from build123d import *


with BuildPart() as part:
    # Sketch6 → Revolve1 (revolve)
    with BuildSketch(Plane.XY, mode=Mode.PRIVATE) as revolve1_sk:
        with BuildLine():
            Line((50.8, 22.53035676), (50.8, 6.35))
            Line((50.8, 6.35), (53.975, 6.35))
            Line((53.975, 6.35), (53.975, 20.227565916))
            add(Edge.make_bspline(
                [(53.975, 20.227565916), (54.291634879, 20.330430839), (55.162475518, 20.612719168), (56.636149311, 21.087725347), (58.867170376, 21.80102074), (61.522421046, 22.638682883), (64.736507837, 23.637812157), (68.023541536, 24.646609183), (72.39438926, 25.969741612), (77.802325895, 27.573199633), (84.37229967, 29.477097548), (93.118193973, 31.954107645), (108.466778526, 36.165197289), (130.491628823, 41.875745108), (165.870302673, 50.489926314), (210.303076361, 60.449379541), (281.693068548, 75.067985253), (371.347473816, 91.310304544), (479.374979471, 108.229836311), (569.684892552, 120.376775068), (642.076792345, 128.912483065), (696.438363769, 134.692640498), (750.863527692, 139.800693107), (796.267539796, 143.42521879), (832.617797313, 145.860290015), (859.890749047, 147.416222506), (882.628689993, 148.436275801), (898.53412358, 148.946546098), (907.62769622, 149.150954449), (912.14731785, 149.217348506), (914.4107585, 149.225018228)],
                knots=[0.06148136, 0.06148136, 0.06148136, 0.06148136, 0.06256458, 0.064402689, 0.066240798, 0.069917015, 0.073593232, 0.07726945, 0.080945667, 0.088298102, 0.095650536, 0.103002971, 0.11770784, 0.147117579, 0.176527318, 0.235346795, 0.294166272, 0.411805227, 0.529444182, 0.647083136, 0.705902613, 0.764722091, 0.823541568, 0.882361045, 0.911770784, 0.941180523, 0.970590261, 0.985295131, 0.992647565, 1, 1, 1, 1], degree=3))
            Line((914.4107585, 149.225018228), (914.4107585, 146.05))
            Line((914.4107585, 146.05), (1066.8, 146.05))
            Line((1066.8, 146.05), (1066.8, 149.225))
            Line((1066.8, 149.225), (965.2, 149.225))
            Line((965.2, 149.225), (965.2, 152.4))
            Line((965.2, 152.4), (914.4, 152.4))
            add(Edge.make_bspline(
                [(50.8, 22.53035676), (51.62596102, 22.801930188), (53.247366667, 23.331443773), (57.113810342, 24.581671091), (62.137627853, 26.163245596), (68.472923462, 28.113411094), (76.389796689, 30.474842786), (85.386033894, 33.081102875), (95.241355255, 35.841520364), (106.104903016, 38.788706559), (117.812200959, 41.867831442), (130.423899043, 45.08497442), (143.907449646, 48.417167108), (158.285989872, 51.860839853), (172.682057827, 55.208017205), (187.101006341, 58.468808185), (201.536340401, 61.648015415), (215.98908439, 64.751824582), (234.073297096, 68.542392147), (255.802551989, 72.956576003), (281.189453131, 77.92470015), (306.614812158, 82.692611325), (328.432361696, 86.646151134), (350.268122203, 90.497714312), (372.121192631, 94.250003895), (397.640090518, 98.488121242), (426.834492226, 103.147632175), (456.056824987, 107.628600482), (485.305388678, 111.934967932), (514.578772116, 116.069226586), (543.875783343, 120.032588186), (573.19542697, 123.82488003), (602.536868801, 127.444739672), (631.89942018, 130.889153604), (661.282519219, 134.153873932), (698.036524214, 138.001817701), (742.180870702, 142.229994267), (786.373789985, 145.926990276), (830.615211008, 148.98950394), (864.145536025, 150.817451898), (884.93243709, 151.702539519), (900.347440379, 152.177178216), (908.376949057, 152.340862845), (912.39222778, 152.393196617), (914.4, 152.4)],
                knots=[0.058888363, 0.058888363, 0.058888363, 0.058888363, 0.058888363, 0.06286181, 0.066835256, 0.074782149, 0.082729042, 0.090675935, 0.102752696, 0.114829458, 0.126906219, 0.138982981, 0.154876753, 0.170770526, 0.186664299, 0.202558071, 0.218451844, 0.234345618, 0.250239391, 0.266133165, 0.297920711, 0.329708258, 0.361495805, 0.377389579, 0.393283353, 0.4250709, 0.456858447, 0.488645994, 0.52043354, 0.552221087, 0.584008633, 0.615796181, 0.647583729, 0.679371276, 0.711158823, 0.74294637, 0.774733917, 0.838309011, 0.901884107, 0.933671654, 0.965459201, 0.9827296, 0.9913648, 1, 1, 1, 1, 1], degree=4))
        make_face()
    revolve(revolve1_sk.sketch.rotate(Axis((-61.64472501, 0, 0), (1, 0, 0)), 90), axis=Axis((-61.64472501, 0, 0), (1, 0, 0)))


solid = part.part
Input: part model. Units: mm. Frame: model coordinates. A direction names the side the tool comes from. Coordinates: 2 decimals unless noted, no trailing zeros. Loops run counter-clockwise (first coordinate to the right, second up) from the corner with the lowest first, then second, coordinate; pieces in that order, holes last. Notation, with made-up numbers: (46, -27) - (50, -27) arc R21 cw to (50, -5) - close; hole circle Ø4 at (-9.5, 64.5). An arc over 180 degrees is marked (long way). Answer in a Markdown table with one row per item. Add a question column.
Item 1: Access query for faces 1 (the cylindrical face through (939.444, 148.776, -33.037)), 2 (the cylindrical face through (1015.289, 145.676, -32.349)). Directions: +Z, -Z, +X, -X, +Y, -Y. A direction counts if a zero-diameter tool reaches every point of the face in a straight line with its end or side. Return the directions, or none.
Item 2: Contact query for flat-ended pins moving along their axis: P1, Ø5, axis at x = 565, z = -80, coming from the -Y side; P2, Ø1, axis at x = 264, y = 11, coming from the +Z side; P3, Ø5, axis at x = 891, z = 40, coming from the +Y side. Output: stop coordinate, or through.
Item 3: Mould query, pull axis X, two halves, no side actions, for faces 3 (the flat face through (53.975, -5, 5)), 4 (the flat face through (914.411, 110, 99)), 5 (the cylindrical face through (991.672, 129.571, 67.393)). Classes: released by +X, released by -X, zero draft, split by the parting line, or undercut.
Item 4: Section query A-A on x = 930. Return the cut outline in (y, z).
Item 5: Line query: line 1 along Y through (x, z) = (1036, 0) (3 decimals); line 2 along Y through (x, z) = (806, 20); line 3 along Z through (x, y) = (372, -3.5). Output: solid intervals per line, ascending. Write a range as [from, to].
Recorded:
| question | item | result |
|---|---|---|
| 1 | face 1 | +X, -X |
| 1 | face 2 | +X |
| 2 | P1 | y = -95.23 |
| 2 | P2 | z = 73.85 |
| 2 | P3 | y = 147.18 |
| 3 | face 3 | released by +X |
| 3 | face 4 | undercut |
| 3 | face 5 | zero draft |
| 4 | outline | circle Ø304.8 at (0, 0); hole circle Ø292.1 at (0, 0) |
| 5 | line 1 | [-149.225, -146.05], [146.05, 149.225] |
| 5 | line 2 | [-145.86, -142.65], [142.65, 145.86] |
| 5 | line 3 | [-94.13, -90.91], [90.91, 94.13] |
